Input: part model. Units: mm. Frame: model coordinates. A direction names the side the tool comes from. Coordinates: 2 decimals unless noted, no trailing zeros. Loops run counter-clockwise (first coordinate to the right, second up) from the corner with the lowest first, then second, coordinate; pieces in that order, holes last.
Item 1: Pull-direction query (X, two-part tool) for faces 3 (the flat face through (101.5, 0, 9)), 4 (the cylindrical face through (-89.917, -21.037, 8.874)), 5 (the cylindrical face through (-90.037, 20.917, 8.874)), 6 (the flat face through (-1, -32.5, 9)); classes: released by +X, released by -X, zero draft, split by the parting line, or undercut.
Item 2: Section C-C on x = -43. Return loops of the section in (y, z).
Item 3: Section A-A on y = -15. Return loops of the section in (x, z), and give its area (3 significant figures).
Item 4: Reachability of faces 1 (the flat face through (7, 27, 18)), 2 (the flat face through (1, -26.5, 9)) from +Z, -Z, +X, -X, +Y, -Y: full face, straight path, thin tool, end or side. Return the list, or none.
Item 5: Contact query for a flat-ended pin moving along its axis: P1, Ø4.5, axis at x = 94.75, y = -25.75, coming from the +Z side. Output: stop coordinate, or through.
Item 6: Ray query, line 1 along X through (y, z) = (25.5, 15.25); line 2 along Y through (x, z) = (23.5, 11.25); line 3 along X through (y, z) = (-2.5, 8). Return the intervals inside material, ascending.
Item 7: Section B-B on z = 13.75. Return loops of the section in (x, y), and give its area (3 significant figures).
```python
from build123d import *

# Parameters (mm, degrees)
F0_R     = 1.75
F1_DEPTH = 18


with BuildPart() as f1:
    # F0 (on Top) → F1 (new body)
    with BuildSketch(Plane.XY):
        with BuildLine():
            Line((-94.75, -32.5), (94.75, -32.5))
            ThreePointArc((94.75, -32.5), (99.522971, -30.522971), (101.5, -25.75))
            Line((101.5, -25.75), (101.5, 25.75))
            ThreePointArc((101.5, 25.75), (99.522971, 30.522971), (94.75, 32.5))
            Line((94.75, 32.5), (-94.75, 32.5))
            ThreePointArc((-94.75, 32.5), (-99.522971, 30.522971), (-101.5, 25.75))
            Line((-101.5, 25.75), (-101.5, -25.75))
            ThreePointArc((-101.5, -25.75), (-99.522971, -30.522971), (-94.75, -32.5))
        make_face()
        with Locations((-94.75, -25.75)):
            Circle(F0_R, mode=Mode.SUBTRACT)
        with Locations((94.75, -25.75)):
            Circle(F0_R, mode=Mode.SUBTRACT)
        with Locations((-94.75, 25.75)):
            Circle(F0_R, mode=Mode.SUBTRACT)
        with BuildLine():
            Line((6.708204, 26.5), (88.041796, 26.5))
            ThreePointArc((88.041796, 26.5), (89.977029, 20.977029), (95.5, 19.041796))
            Line((95.5, 19.041796), (95.5, -19.041796))
            ThreePointArc((95.5, -19.041796), (89.977029, -20.977029), (88.041796, -26.5))
            Line((88.041796, -26.5), (6.708204, -26.5))
            Line((6.708204, -26.5), (-88.041796, -26.5))
            ThreePointArc((-88.041796, -26.5), (-89.977029, -20.977029), (-95.5, -19.041796))
            Line((-95.5, -19.041796), (-95.5, 19.041796))
            ThreePointArc((-95.5, 19.041796), (-89.977029, 20.977029), (-88.041796, 26.5))
            Line((-88.041796, 26.5), (6.708204, 26.5))
        make_face(mode=Mode.SUBTRACT)
        with Locations((94.75, 25.75)):
            Circle(F0_R, mode=Mode.SUBTRACT)
    extrude(amount=F1_DEPTH)


solid = f1.part
```
Results found:
1. face 3: released by +X
1. face 4: undercut
1. face 5: undercut
1. face 6: zero draft
2. outline: (-32.5, 0) - (-26.5, 0) - (-26.5, 18) - (-32.5, 18) - close; (26.5, 0) - (32.5, 0) - (32.5, 18) - (26.5, 18) - close
3. outline: (-101.5, 0) - (-95.5, 0) - (-95.5, 18) - (-101.5, 18) - close; (95.5, 0) - (101.5, 0) - (101.5, 18) - (95.5, 18) - close
3. area: 216 mm2
4. face 1: +Z, +X, -X, +Y, -Y
4. face 2: +Z, -Z
5. P1: stops at z = 18
6. line 1: x = -101.5 to -96.48, -93.02 to -88, 88 to 93.02, 96.48 to 101.5
6. line 2: y = -32.5 to -26.5, 26.5 to 32.5
6. line 3: x = -101.5 to -95.5, 95.5 to 101.5
7. outline: (-101.5, -25.75) arc R6.75 ccw to (-94.75, -32.5) - (94.75, -32.5) arc R6.75 ccw to (101.5, -25.75) - (101.5, 25.75) arc R6.75 ccw to (94.75, 32.5) - (-94.75, 32.5) arc R6.75 ccw to (-101.5, 25.75) - close; hole circle Ø3.5 at (-94.75, -25.75); hole circle Ø3.5 at (-94.75, 25.75); hole (-95.5, -19.04) arc R6.75 cw to (-88.04, -26.5) - (88.04, -26.5) arc R6.75 cw to (95.5, -19.04) - (95.5, 19.04) arc R6.75 cw to (88.04, 26.5) - (-88.04, 26.5) arc R6.75 cw to (-95.5, 19.04) - close; hole circle Ø3.5 at (94.75, -25.75); hole circle Ø3.5 at (94.75, 25.75)
7. area: 3,180 mm2
